Solid Edge part; units mm, degrees
sketch "Sketch1" plane through (0, 0, 0) normal (1, 0, 0) x (0, 1, 0)
  line L0 (-39.3116, 40.5502) -> (-41.8516, 40.5502)
  line L1 (-16.4516, 40.5502) -> (-18.9916, 40.5502)
  arc A0 (-18.9916, 40.5502) -> (-39.3116, 40.5502) centre (-29.1516, 40.5502) cw
  arc A1 (-41.8516, 40.5502) -> (-16.4516, 40.5502) centre (-29.1516, 40.5502) ccw
extrude "Protrusion1" add sketch "Sketch1" along normal mid plane 203.2
sketch "Sketch2" plane through (0, -17.7216, 0) normal (0, -1, 0) x (1, 0, 0)
  circle A0 centre (63.5, 40.5502) radius 4.6933
  circle A1 centre (-63.5, 40.5502) radius 4.6933
extrude "Protrusion2" add sketch "Sketch2" along normal mid plane 2.54
sketch "Sketch3" plane through (63.5, -16.4516, 40.5502) normal (0, 1, 0) x (-1, 0, 0)
  circle A0 centre (127, 0) radius 2.2225
  circle A1 centre (0, 0) radius 2.2225
extrude "Cutout1" cut sketch "Sketch3" against normal up to vertex (12.7 mm away)
properties material "ALUMINUM"
Source: CAD feature listing. Evaluate the final solid. Frame: model axes, mm. A direction names the side the tool comes from. Round coordinates to 2 decimals unless told otherwise and drop trailing zeros. Order: outer loops, then holes, each group sorted by start corner. A loop starts at its lowest first (then second) coordinate and runs counter-clockwise, first axis right, second up. Notation, with made-up numbers: (1, -32) - (30, -32) arc R22 cw to (30, -25) - close; hole circle Ø5 at (88.5, -11). An arc over 180 degrees is marked (long way). Use a Markdown table: item, result. Add a question column.
1. Set-up query: faces 1 (the cylindrical face through (-63.02, -17.83, 38.38)), 2 (the flat face through (64, -18.992, 43)), 3 (the cylindrical face through (63.397, -16.808, 35.858)). Return all of +Z, -Z, +X, -X, +Y, -Y with unobstructed straight access to the full face (end or side cutting, diameter ignored); none if empty.
2. Section query C-C (y = -29.5). Return the cut outline in (x, z), then the cut area to 3 significant figures.
3. First-contact query: pin 1 (10 mm diameter, centred on x = -6.5, z = 32, fed in from +Y); pin 2 (3 mm diameter, centred on x = 14, y = -17.5, fed in from +Z); pin 3 (3 mm diameter, centred on x = -11.5, y = -35, fed in from -Z); pin 4 (10 mm diameter, centred on x = 55, y = -27, fed in from -Z). Flat tips, straight axial feed; report the tip coordinate or a pass-through.
4. Section query A-A (x = 63.5). Return the cut outline in (y, z).
5. Section query B-B (x = 27.5). Return the cut outline in (y, z).
6. Mould query, pull axis Y, two halves, no side actions, for faces 4 (the flat face through (-63, -18.992, 43)), 5 (the flat face through (-66, -16.452, 40)), 6 (the cylindrical face through (-1.422, -28.928, 30.393)), 7 (the cylindrical face through (63.603, -17.739, 45.242)). Classes: +Y half, -Y half, draft (parallel to the pull), parting line (faces both ways), or undercut.
7. Line query: probe 1 along Y at (x, z) = (-86, 40.25); probe 2 along Y at (x, z) = (93, 40.5); probe 3 along Z at (x, y) = (63.5, -17.35). Output: solid intervals per line, ascending.
Derived:
| question | item | result |
|---|---|---|
| 1 | face 1 | +Y |
| 1 | face 2 | +Z, +X, -X, -Y |
| 1 | face 3 | -Z, +Y |
| 2 | outline | (-101.6, 27.85) - (101.6, 27.85) - (101.6, 30.4) - (-101.6, 30.4) - close |
| 2 | area | 516 mm2 |
| 3 | pin 1 | y = -16.96 |
| 3 | pin 2 | z = 40.55 |
| 3 | pin 3 | z = 28.62 |
| 3 | pin 4 | z = 27.85 |
| 4 | outline | (-41.85, 40.55) arc R12.7 ccw to (-17.35, 35.86) - (-16.45, 35.86) - (-16.45, 38.33) - (-19.24, 38.33) arc R10.16 cw to (-39.31, 40.55) - close; (-18.99, 42.77) - (-16.45, 42.77) - (-16.45, 45.24) - (-18.99, 45.24) - close |
| 5 | outline | (-41.85, 40.55) arc R12.7 ccw to (-16.45, 40.55) - (-18.99, 40.55) arc R10.16 cw to (-39.31, 40.55) - close |
| 6 | face 4 | -Y half |
| 6 | face 5 | +Y half |
| 6 | face 6 | undercut |
| 6 | face 7 | draft |
| 7 | probe 1 | -41.85 to -39.31, -19 to -16.46 |
| 7 | probe 2 | -41.85 to -39.31, -18.99 to -16.45 |
| 7 | probe 3 | 35.86 to 38.33, 42.77 to 45.24 |
